from build123d import *

# Parameters (mm, degrees)
SKETCH_1_W                  = 130
SKETCH_1_H                  = 125
SKETCH_1_R                  = 6
EXTRUDE_1_DEPTH             = 60
HOLE_WIZARD_12_0_12_1_D     = 12
HOLE_WIZARD_12_0_12_1_DEPTH = 30
HOLE_WIZARD_12_0_12_1_TIP   = 3.605163714
HOLE_WIZARD_12_0_12_2_D     = 12
HOLE_WIZARD_12_0_12_2_DEPTH = 12
HOLE_WIZARD_12_0_12_2_TIP   = 3.605163714
HOLE_WIZARD_4_0_4_1_D       = 4
HOLE_WIZARD_M10_2_D         = 8.5
HOLE_WIZARD_M10_2_DEPTH     = 14
HOLE_WIZARD_M10_2_TIP       = 2.553657631
HOLE_WIZARD_M5_2_D          = 4.2
HOLE_WIZARD_M5_2_DEPTH      = 14
HOLE_WIZARD_M5_2_TIP        = 1.2618073
HOLE_WIZARD_8_0_8_2_D       = 8
HOLE_WIZARD_8_0_8_2_DEPTH   = 52
HOLE_WIZARD_8_0_8_2_TIP     = 2.403442476
HOLE_WIZARD_M10_3_D         = 8.5
HOLE_WIZARD_M10_3_DEPTH     = 8
HOLE_WIZARD_M10_3_TIP       = 2.553657631
HOLE_WIZARD_8_0_8_3_D       = 8
HOLE_WIZARD_8_0_8_3_DEPTH   = 86
HOLE_WIZARD_8_0_8_3_TIP     = 2.403442476
SKETCH_3_R                  = 2
CUT_EXTRUDE_1_DEPTH         = 39
SKETCH_31_R                 = 3
CUT_EXTRUDE_2_DEPTH         = 60
SKETCH_32_R                 = 2
CUT_EXTRUDE_3_DEPTH         = 69
HOLE_WIZARD_M10_4_D         = 8.5
HOLE_WIZARD_M10_4_DEPTH     = 13.5
HOLE_WIZARD_M10_4_TIP       = 2.553657631


with BuildPart() as part:
    # 草图1 → 凸台-拉伸1 (new body)
    with BuildSketch(Plane.XY):
        Rectangle(SKETCH_1_W, SKETCH_1_H)
        with Locations((-55, -52.5)):
            Circle(SKETCH_1_R, mode=Mode.SUBTRACT)
        with Locations((55, -52.5)):
            Circle(SKETCH_1_R, mode=Mode.SUBTRACT)
        with Locations((55, 52.5)):
            Circle(SKETCH_1_R, mode=Mode.SUBTRACT)
        with Locations((-55, 52.5)):
            Circle(SKETCH_1_R, mode=Mode.SUBTRACT)
    extrude(amount=-EXTRUDE_1_DEPTH)

    # Ø12.0 (12) 直径孔1
    with Locations(Plane(origin=(5, -7.5, 0), x_dir=(1, 0, 0), z_dir=(0, 0, 1))):
        with Locations((0, 0)):
            Hole(HOLE_WIZARD_12_0_12_1_D / 2, depth=HOLE_WIZARD_12_0_12_1_DEPTH)
            with Locations((0, 0, -(HOLE_WIZARD_12_0_12_1_DEPTH + HOLE_WIZARD_12_0_12_1_TIP / 2))):  # 118° drill point
                Cone(0, HOLE_WIZARD_12_0_12_1_D / 2, HOLE_WIZARD_12_0_12_1_TIP, mode=Mode.SUBTRACT)

    # Ø12.0 (12) 直径孔2
    with Locations(Plane(origin=(-35, -27.5, 0), x_dir=(1, 0, 0), z_dir=(0, 0, 1))):
        with Locations((0, 0)):
            Hole(HOLE_WIZARD_12_0_12_2_D / 2, depth=HOLE_WIZARD_12_0_12_2_DEPTH)
            with Locations((0, 0, -(HOLE_WIZARD_12_0_12_2_DEPTH + HOLE_WIZARD_12_0_12_2_TIP / 2))):  # 118° drill point
                Cone(0, HOLE_WIZARD_12_0_12_2_D / 2, HOLE_WIZARD_12_0_12_2_TIP, mode=Mode.SUBTRACT)

    # Ø4.0 (4) 直径孔1 (through all)
    with Locations(Plane(origin=(0, 62.5, 0), x_dir=(1, 0, 0), z_dir=(0, 1, 0))):
        with Locations((-13, 48), (-31, 30)):
            Hole(HOLE_WIZARD_4_0_4_1_D / 2)

    # M10 螺纹孔2
    with Locations(Plane(origin=(0, -62.5, 0), x_dir=(-1, 0, 0), z_dir=(0, -1, 0))):
        with Locations((31, 30), (13, 48)):
            Hole(HOLE_WIZARD_M10_2_D / 2, depth=HOLE_WIZARD_M10_2_DEPTH)
            with Locations((0, 0, -(HOLE_WIZARD_M10_2_DEPTH + HOLE_WIZARD_M10_2_TIP / 2))):  # 118° drill point
                Cone(0, HOLE_WIZARD_M10_2_D / 2, HOLE_WIZARD_M10_2_TIP, mode=Mode.SUBTRACT)

    # M5 螺纹孔2
    with Locations(Plane(origin=(0, 62.5, 0), x_dir=(1, 0, 0), z_dir=(0, 1, 0))):
        with Locations((-33, 50), (7, 50), (7, 10), (-33, 10)):
            Hole(HOLE_WIZARD_M5_2_D / 2, depth=HOLE_WIZARD_M5_2_DEPTH)
            with Locations((0, 0, -(HOLE_WIZARD_M5_2_DEPTH + HOLE_WIZARD_M5_2_TIP / 2))):  # 118° drill point
                Cone(0, HOLE_WIZARD_M5_2_D / 2, HOLE_WIZARD_M5_2_TIP, mode=Mode.SUBTRACT)

    # Ø8.0 (8) 直径孔2
    with Locations(Plane(origin=(-65, 23.5, -12), x_dir=(0, 0, -1), z_dir=(-1, 0, 0))):
        with Locations((0, 0)):
            Hole(HOLE_WIZARD_8_0_8_2_D / 2, depth=HOLE_WIZARD_8_0_8_2_DEPTH)
            with Locations((0, 0, -(HOLE_WIZARD_8_0_8_2_DEPTH + HOLE_WIZARD_8_0_8_2_TIP / 2))):  # 118° drill point
                Cone(0, HOLE_WIZARD_8_0_8_2_D / 2, HOLE_WIZARD_8_0_8_2_TIP, mode=Mode.SUBTRACT)

    # M10 螺纹孔3
    with Locations(Plane(origin=(-65, 23.5, -12), x_dir=(0, 0, -1), z_dir=(-1, 0, 0))):
        with Locations((0, 0)):
            Hole(HOLE_WIZARD_M10_3_D / 2, depth=HOLE_WIZARD_M10_3_DEPTH)
            with Locations((0, 0, -(HOLE_WIZARD_M10_3_DEPTH + HOLE_WIZARD_M10_3_TIP / 2))):  # 118° drill point
                Cone(0, HOLE_WIZARD_M10_3_D / 2, HOLE_WIZARD_M10_3_TIP, mode=Mode.SUBTRACT)

    # Ø8.0 (8) 直径孔3
    with Locations(Plane(origin=(-35, -62.5, -12), x_dir=(0, 0, -1), z_dir=(0, -1, 0))):
        with Locations((0, 0)):
            Hole(HOLE_WIZARD_8_0_8_3_D / 2, depth=HOLE_WIZARD_8_0_8_3_DEPTH)
            with Locations((0, 0, -(HOLE_WIZARD_8_0_8_3_DEPTH + HOLE_WIZARD_8_0_8_3_TIP / 2))):  # 118° drill point
                Cone(0, HOLE_WIZARD_8_0_8_3_D / 2, HOLE_WIZARD_8_0_8_3_TIP, mode=Mode.SUBTRACT)

    # 草图3 → 切除-拉伸1 (cut)
    with BuildSketch(Plane(origin=(0, 62.5, 0), x_dir=(1, 0, 0), z_dir=(0, 1, 0))):
        with Locations((-13, 12)):
            Circle(SKETCH_3_R)
    extrude(amount=-CUT_EXTRUDE_1_DEPTH, mode=Mode.SUBTRACT)

    # 草图31 → 切除-拉伸2 (cut)
    with BuildSketch(Plane(origin=(65, 0, 0), x_dir=(0, 0, -1), z_dir=(1, 0, 0))):
        with Locations((30, -7.5)):
            Circle(SKETCH_31_R)
    extrude(amount=-CUT_EXTRUDE_2_DEPTH, mode=Mode.SUBTRACT)

    # 草图32 → 切除-拉伸3 (cut)
    with BuildSketch(Plane(origin=(0, 62.5, 0), x_dir=(1, 0, 0), z_dir=(0, 1, 0))):
        with Locations((5, 30)):
            Circle(SKETCH_32_R)
    extrude(amount=-CUT_EXTRUDE_3_DEPTH, mode=Mode.SUBTRACT)

    # M10 螺纹孔4
    with Locations(Plane(origin=(-35, -62.5, -12), x_dir=(0, 0, -1), z_dir=(0, -1, 0))):
        with Locations((0, 0)):
            Hole(HOLE_WIZARD_M10_4_D / 2, depth=HOLE_WIZARD_M10_4_DEPTH)
            with Locations((0, 0, -(HOLE_WIZARD_M10_4_DEPTH + HOLE_WIZARD_M10_4_TIP / 2))):  # 118° drill point
                Cone(0, HOLE_WIZARD_M10_4_D / 2, HOLE_WIZARD_M10_4_TIP, mode=Mode.SUBTRACT)


solid = part.part
Input: part model. Units: mm. Frame: model coordinates. A direction names the side the tool comes from. Give positions to 0.01 mm unless a question says otherwise; leave off trailing zeros. Loops run counter-clockwise (first coordinate to the right, second up) from the corner with the lowest first, then second, coordinate; pieces in that order, holes last. Notation, with made-up numbers: (23.5, -38.5) -> (74.5, -38.5) arc R9 ccw to (74.5, -21.5) -> close; hole circle Ø2 at (5, 65). An arc over 180 degrees is marked (long way). Answer as a JSON object with one key per item and string values. Group by question number.
Item 1: Cut plane C-C, the plane x = 55. Return the cut outline in (y, z), and give its area (3 significant figures).
Item 2: Pin query (flat end, axial travel): P1, Ø9.5, axis at x = 5, y = -7.5, coming from the +Z side; P2, Ø2.5, axis at x = -31, z = -30, coming from the -Y side; P3, Ø2.5, axis at x = -33, z = -50, coming from the +Y side; P4, Ø5, axis at x = -35, z = -12, coming from the -Y side. Return the tip coordinate at first contact, or that it passes through.
Item 3: Cut plane B-B, the plane z = -38. Return the cut outline in (x, y).
Item 4: Pull-direction query (X, two-part tool) for faces 1 (the cylindrical face through (-30.9, 55.4, -10.09)), 2 (the conical face through (-11.28, 22.37, -11.85)), 3 (the flat face through (65, -1, -30)), 4 (the conical face through (-33.27, 47.46, -10.25)); classes: released by +X, released by -X, zero draft, split by the parting line, or undercut.
Item 5: Reachability of faces 5 (the cylindrical face through (-11.04, -55.4, -44.23)), 6 (the cylindrical face through (-29.006, -27.236, -6.084)), 7 (the flat face through (-65, -1, -30)), 8 (the cylindrical face through (7.273, 55.402, -12.082)), 9 (the cylindrical face through (-60.94, 27.65, -12.92)) from +Z, -Z, +X, -X, +Y, -Y: full face, straight path, thin tool, end or side. Return the list, or none.
Item 6: Line query: probe 1 along Z at (x, y) = (-13, -56); probe 2 along X at (y, z) = (-56.5, -48); probe 3 along X at (y, z) = (-56.5, -23). Output: solid intervals per line, ascending.
Item 7: Cut plane D-D, the plane y = -30. State how many separate pieces and enclosed holes the cut face has, and give its area (3 significant figures).
Item 8: Cut plane A-A, the plane x = -55. Return the cut outline in (y, z), and give its area (3 significant figures).
Checks:
{
 "1": {"outline": "(-62.5, -60) -> (-58.5, -60) -> (-58.5, 0) -> (-62.5, 0) -> close; (-46.5, -60) -> (46.5, -60) -> (46.5, 0) -> (-46.5, 0) -> close; (58.5, -60) -> (62.5, -60) -> (62.5, 0) -> (58.5, 0) -> close; hole circle Ø6 at (-7.5, -30)", "area": "6,030 mm²"},
 "2": {"P1": "stops at z = -30.75", "P2": "passes through", "P3": "stops at y = 47.99", "P4": "stops at y = 26.62"},
 "3": {"outline": "(-65, -62.5) -> (65, -62.5) -> (65, 62.5) -> (-65, 62.5) -> close; hole circle Ø12 at (-55, -52.5); hole circle Ø12 at (-55, 52.5); hole circle Ø12 at (55, -52.5); hole circle Ø12 at (55, 52.5)"},
 "4": {"face 1": "undercut", "face 2": "released by -X", "face 3": "released by +X", "face 4": "undercut"},
 "5": {"face 5": "-Y", "face 6": "+Z", "face 7": "+Z, -Z, -X, +Y, -Y", "face 8": "+Y", "face 9": "-X"},
 "6": {"probe 1": "z = -60 to -52.25, -43.75 to 0", "probe 2": "x = -65 to -59.47, -50.53 to -17.25, -8.75 to 50.53, 59.47 to 65", "probe 3": "x = -65 to -59.47, -50.53 to 50.53, 59.47 to 65"},
 "7": {"separate pieces": "1", "enclosed holes": "2", "area": "7,620 mm²"},
 "8": {"outline": "(-62.5, -60) -> (-58.5, -60) -> (-58.5, 0) -> (-62.5, 0) -> close; (-46.5, -60) -> (46.5, -60) -> (46.5, 0) -> (-46.5, 0) -> close; (58.5, -60) -> (62.5, -60) -> (62.5, 0) -> (58.5, 0) -> close; hole circle Ø8 at (23.5, -12)", "area": "6,010 mm²"}
}
